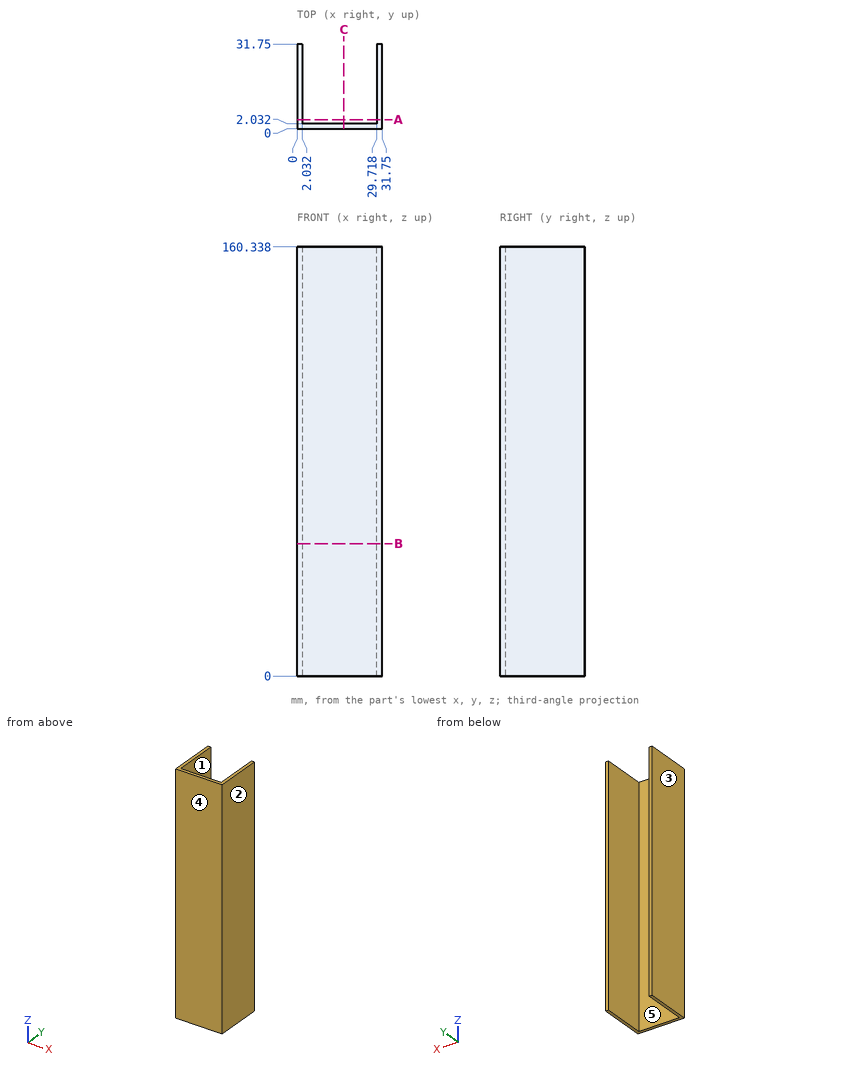
Geometry: see drawing. Coordinates: mm, zero at the bounding-box minimum. A direction names the side the tool comes from. Round coordinates to 2 decimals unless told otherwise and drop trailing zeros. Write each loop counter-clockwise with the first axis right and the second up, starting at its lowest first coordinate (ties: lowest second). Pieces come first, ordered by that corner, then holes.
Item 1: Material intervals for L1, parallel to X at y = 21, z = 11; L2, parallel to Y at x = 26.5, z = 52, sorted ascending.
Item 2: Pin query (flat end, axial travel): P1, Ø6, axis at x = 24, y = 14, coming from the -Z side; P2, Ø8.5, axis at x = 10, z = 75.5, coming from the +Y side. Return the tip coordinate at first contact, or that it passes through.
Item 3: Mould query, pull axis X, two halves, no side actions, for the marked faces 1, 2 and 3. Classes: +X half, -X half, draft (parallel to the pull), parting line (faces both ways), or undercut.
Item 4: Section query B-B (z = 49.5). Return loops of the section in (x, y).
Item 5: Section query C-C (x = 17.5). Return loops of the section in (y, z).
Item 6: Set-up query: the marked faces 4 and 5. Return all of +Z, -Z, +X, -X, +Y, -Y with unobstructed straight access to the full face (end or side cutting, diameter ignored); none if empty.
Item 7: Section query A-A (y = 3.5). Return loops of the section in (x, z).
Completed:
1. L1: x = 0 to 2.03, 29.72 to 31.75
1. L2: y = 0 to 2.03
2. P1: passes through
2. P2: stops at y = 2.03
3. face 1: undercut
3. face 2: +X half
3. face 3: -X half
4. outline: (0, 0) - (31.75, 0) - (31.75, 31.75) - (29.72, 31.75) - (29.72, 2.03) - (2.03, 2.03) - (2.03, 31.75) - (0, 31.75) - close
5. outline: (0, 0) - (2.03, 0) - (2.03, 160.34) - (0, 160.34) - close
6. face 4: +Z, -Z, +X, -X, -Y
6. face 5: +Z, -Z, +Y
7. outline: (0, 0) - (2.03, 0) - (2.03, 160.34) - (0, 160.34) - close; (29.72, 0) - (31.75, 0) - (31.75, 160.34) - (29.72, 160.34) - close
